The listing builds one solid part. Answer for the finished solid, in the listing's coordinates (mm). Face numbers are marked on the shaded views. A direction names the side the tool comes from. Round coordinates to 2 decimals unless told otherwise and drop trailing zeros. Order: outer loops, then holes, each group sorted by start corner. A loop starts at its lowest first (then second) coordinate and runs counter-clockwise, first axis right, second up. Notation, with made-up numbers: (64.25, -30.5) - (81.25, -30.5) arc R23 ccw to (81.25, -7.5) - close; hole circle Ø4 at (-1, 67). An arc over 180 degrees is marked (long way). Write item = value, one per line.
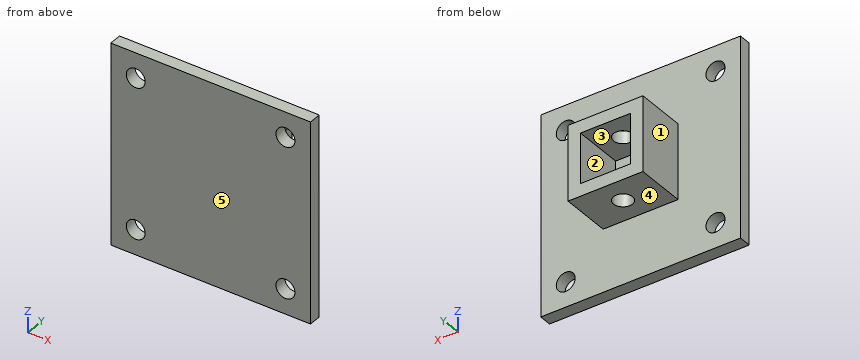
from build123d import *

# Parameters (mm, degrees)
SKETCH1_W               = 101.6
SKETCH1_H               = 101.6
BOSS_EXTRUDE1_DEPTH     = 6.35
SKETCH2_W               = 38.1
SKETCH2_H               = 38.1
SKETCH2_W_2             = 25.4
SKETCH2_H_2             = 25.4
BOSS_EXTRUDE2_DEPTH     = 25.4
SKETCH3_R               = 4.826
CUT_EXTRUDE1_DEPTH      = 32.75
CUT_EXTRUDE1_DEPTH_BACK = 70.85
SKETCH4_R               = 4.826
CUT_EXTRUDE2_DEPTH      = 25.4


with BuildPart() as part:
    # Sketch1 → Boss-Extrude1 (new body)
    with BuildSketch(Plane(origin=(0, 0, 0), x_dir=(1, 0, 0), z_dir=(0, 1, 0))):
        Rectangle(SKETCH1_W, SKETCH1_H)
    extrude(amount=BOSS_EXTRUDE1_DEPTH)

    # Sketch2 → Boss-Extrude2 (add)
    with BuildSketch(Plane(origin=(0, 6.35, 0), x_dir=(1, 0, 0), z_dir=(0, 1, 0))):
        Rectangle(SKETCH2_W, SKETCH2_H)
        Rectangle(SKETCH2_W_2, SKETCH2_H_2, mode=Mode.SUBTRACT)
    extrude(amount=BOSS_EXTRUDE2_DEPTH)

    # Sketch3 → Cut-Extrude1 (cut, two sides)
    with BuildSketch(Plane.XY.offset(19.05)) as cut_extrude1_sk:
        with Locations((0, 19.05)):
            Circle(SKETCH3_R)
    extrude(amount=CUT_EXTRUDE1_DEPTH, mode=Mode.SUBTRACT)
    extrude(cut_extrude1_sk.sketch, amount=-CUT_EXTRUDE1_DEPTH_BACK, mode=Mode.SUBTRACT)

    # Sketch4 → Cut-Extrude2 (cut)
    with BuildSketch(Plane(origin=(0, 6.35, 0), x_dir=(1, 0, 0), z_dir=(0, 1, 0))):
        with Locations((-38.1, 38.1)):
            Circle(SKETCH4_R)
        with Locations((38.1, 38.1)):
            Circle(SKETCH4_R)
        with Locations((38.1, -38.1)):
            Circle(SKETCH4_R)
        with Locations((-38.1, -38.1)):
            Circle(SKETCH4_R)
    extrude(amount=-CUT_EXTRUDE2_DEPTH, mode=Mode.SUBTRACT)


solid = part.part
Q1. Find the intervals of material crossed by line 1 (Z direction, x = -38.1, y = 4.25); line 2 (Z direction, x = 8, y = 25), in increasing order. Write a range as from..to.
Model answer:
line_1 = -50.8..-42.93, -33.27..33.27, 42.93..50.8
line_2 = -19.05..-12.7, 12.7..19.05
Q2. Flat-ended cylindrical pins translate along their axes: P1, Ø1.5, axis at y = 11, z = -15.5, coming from the +X side; P2, Ø7.5, axis at x = 1.5, y = 18.5, coming from the +Z side; P3, Ø11, axis at x = -38.1, z = 38.1, coming from the +Y side. Find the tip coordinate at first contact, or state that the pin passes through.
Model answer:
P1 = 19.05
P2 = 19.05
P3 = 6.35
Q3. Section C-C on x = 0 is taken. Determine the outline of the cut face in (y, z), then the cut area to 3 significant figures.
Model answer:
outline = (0, -50.8) - (6.35, -50.8) - (6.35, -19.05) - (14.22, -19.05) - (14.22, -12.7) - (6.35, -12.7) - (6.35, 12.7) - (14.22, 12.7) - (14.22, 19.05) - (6.35, 19.05) - (6.35, 50.8) - (0, 50.8) - close; (23.88, -19.05) - (31.75, -19.05) - (31.75, -12.7) - (23.88, -12.7) - close; (23.88, 12.7) - (31.75, 12.7) - (31.75, 19.05) - (23.88, 19.05) - close
area = 845 mm^2
Q4. Section D-D on y = 16.5 is taken. Determine the outline of the cut face in (x, z).
Model answer:
outline = (-19.05, -19.05) - (-4.1, -19.05) - (-4.1, -12.7) - (-12.7, -12.7) - (-12.7, 12.7) - (-4.1, 12.7) - (-4.1, 19.05) - (-19.05, 19.05) - close; (4.1, -19.05) - (19.05, -19.05) - (19.05, 19.05) - (4.1, 19.05) - (4.1, 12.7) - (12.7, 12.7) - (12.7, -12.7) - (4.1, -12.7) - close
Q5. Determine the mould class of the marked faces 3, 4 and 5 for opening direction Z: released by +Z, released by -Z, zero draft, split by the parting line, or undercut.
Model answer:
face_3 = undercut
face_4 = released by -Z
face_5 = zero draft
Q6. For the marked faces 1 and 2, determine the directions among +Z, -Z, +X, -X, +Y, -Y from which every point of the face is accessible in a straight line to the end or side of a thin tool.
Model answer:
face_1 = +Z, -Z, -X, +Y
face_2 = +Y
Q7. Section A-A on z = -38.1 is taken. Determine the outline of the cut face in (x, y).
Model answer:
outline = (-50.8, 0) - (-42.93, 0) - (-42.93, 6.35) - (-50.8, 6.35) - close; (-33.27, 0) - (33.27, 0) - (33.27, 6.35) - (-33.27, 6.35) - close; (42.93, 0) - (50.8, 0) - (50.8, 6.35) - (42.93, 6.35) - close
Q8. Section B-B on y = 28 is taken. Determine the outline of the cut face in (x, z).
Model answer:
outline = (-19.05, -19.05) - (19.05, -19.05) - (19.05, 19.05) - (-19.05, 19.05) - close; hole (-12.7, -12.7) - (12.7, -12.7) - (12.7, 12.7) - (-12.7, 12.7) - close
